from build123d import *

# Parameters (mm, degrees)
BOSS_EXTRU_2_DEPTH                 = 10
CONG_1_R                           = 0.45
R_P_TITION_CIRCULAIRE1_COUNT       = 8
R_P_TITION_CIRCULAIRE1_ANGLE       = 210
CONG_1_OF_R_P_TITION_CIRCULAIRE1_R = 0.45
ESQUISSE5_R                        = 7.125
BOSS_EXTRU_4_DEPTH                 = 10
ENL_V_MAT_EXTRU_3_DEPTH            = 11
ESQUISSE3_R                        = 1.6
ENL_V_MAT_EXTRU_4_DEPTH            = 11
ESQUISSE8_R                        = 1.6
ENL_V_MAT_EXTRU_5_DEPTH            = 11


with BuildPart() as part:
    # Esquisse1 → Boss.-Extru.2 (new body)
    with BuildSketch(Plane.XY):
        with BuildLine():
            Line((0, 0), (6.882221512, 1.844085696))
            ThreePointArc((6.882221512, 1.844085696), (6.988095123, 1.390018544), (7.064044637, 0.92999912))
            Line((7.064044637, 0.92999912), (8.384880781, 1.103890497))
            ThreePointArc((8.384880781, 1.103890497), (9.465680859, 1.068283463), (10.477518694, 0.686732857))
            ThreePointArc((10.477518694, 0.686732857), (10.5, 0), (10.477518694, -0.686732857))
            ThreePointArc((10.477518694, -0.686732857), (9.465680859, -1.068283463), (8.384880781, -1.103890497))
            Line((8.384880781, -1.103890497), (7.064044637, -0.92999912))
            ThreePointArc((7.064044637, -0.92999912), (6.988095123, -1.390018544), (6.882221512, -1.844085696))
            Line((6.882221512, -1.844085696), (0, 0))
        make_face()
    boss_extru_2 = extrude(amount=BOSS_EXTRU_2_DEPTH)

    # Congé1
    cong_1_edges = [part.edges().sort_by_distance(p)[0] for p in [
        (7.064044637, 0.92999912, 5),
        (7.064044637, -0.92999912, 5),
    ]]
    fillet(cong_1_edges, radius=CONG_1_R)

    # Répétition circulaire1: Boss.-Extru.2 ×8 about axis
    r_p_tition_circulaire1_axis = Axis((0, 0, 0), (0, 0, -1))
    for i in range(1, R_P_TITION_CIRCULAIRE1_COUNT):
        add(boss_extru_2.rotate(r_p_tition_circulaire1_axis, i * R_P_TITION_CIRCULAIRE1_ANGLE / (R_P_TITION_CIRCULAIRE1_COUNT - 1)))

    # Congé1 of Répétition circulaire1
    cong_1_of_r_p_tition_circulaire1_edges = [part.edges().sort_by_distance(p)[0] for p in [
        (6.582641669, -2.726619456, 5),
        (5.65264255, -4.337425182, 5),
        (4.337425182, -5.65264255, 5),
        (2.726619456, -6.582641669, 5),
        (0.92999912, -7.064044637, 5),
        (-0.92999912, -7.064044637, 5),
        (-2.726619456, -6.582641669, 5),
        (-4.337425182, -5.65264255, 5),
        (-5.65264255, -4.337425182, 5),
        (-6.582641669, -2.726619456, 5),
        (-7.064044637, -0.92999912, 5),
        (-7.064044637, 0.92999912, 5),
        (-6.582641669, 2.726619456, 5),
        (-5.65264255, 4.337425182, 5),
    ]]
    fillet(cong_1_of_r_p_tition_circulaire1_edges, radius=CONG_1_OF_R_P_TITION_CIRCULAIRE1_R)

    # Esquisse5 → Boss.-Extru.4 (add, through all)
    with BuildSketch(Plane.XY.offset(10)):
        Circle(ESQUISSE5_R)
    extrude(amount=-BOSS_EXTRU_4_DEPTH)

    # Esquisse7 → Enlèv. mat.-Extru.3 (cut, through all)
    with BuildSketch(Plane.XY.offset(10)):
        with BuildLine():
            Line((-3.608929902, 6.143390755), (6.197120353, 3.515867508))
            ThreePointArc((6.197120353, 3.515867508), (1.844085696, 6.882221512), (-3.608929902, 6.143390755))
        make_face()
    extrude(amount=-ENL_V_MAT_EXTRU_3_DEPTH, mode=Mode.SUBTRACT)

    # Esquisse3 → Enlèv. mat.-Extru.4 (cut, through all)
    with BuildSketch(Plane.XY.offset(10)):
        Circle(ESQUISSE3_R)
    extrude(amount=-ENL_V_MAT_EXTRU_4_DEPTH, mode=Mode.SUBTRACT)

    # Esquisse8 → Enlèv. mat.-Extru.5 (cut, through all)
    with BuildSketch(Plane.XY.offset(10)):
        with Locations((-4.330127019, 2.5)):
            Circle(ESQUISSE8_R)
        with Locations((4.330127019, -2.5)):
            Circle(ESQUISSE8_R)
    extrude(amount=-ENL_V_MAT_EXTRU_5_DEPTH, mode=Mode.SUBTRACT)


solid = part.part
Design review of the part built by this model. Coordinates are the model's own, in mm. A direction names the side the tool comes from. Give positions to 0.01 mm unless a question says otherwise; leave off trailing zeros. Loops run counter-clockwise (first coordinate to the right, second up) from the corner with the lowest first, then second, coordinate; pieces in that order, holes last. Notation, with made-up numbers: (-37, 50) -> (-31, 50) arc R19 ccw to (-31, 65) -> close; hole circle Ø6 at (-35.75, -7.5). An arc over 180 degrees is marked (long way). One line per question, with ' | ' between items. Start each with the question number.
(1) We need section D-D (z = 5). State how many separate pieces and enclosed holes the cut face has, and give its area (3 significant figures).
(2) We need section A-A (y = 0). State the section outline as (x, z) points, and give its area (3 significant figures).
(3) For faces 5 (the face through (5.653, -7.649, 4.93)), 6 (the face through (3.818, -8.743, 4.93)), 7 (the face through (9.481, -1.065, 4.93)), 8 (the face through (-5.663, -7.678, 4.93)), list the 3-axis set-ups (+Z, -Z, +X, -X, +Y, -Y) from which the entire face can be reached by the end or side of a thin tool; tool diameter is ignored.
(4) We need section B-B (x = -4). State the section outline as (y, z) points, and give its area (3 significant figures).
(5) Draft analysis for pull direction X (two halves, no side actions). For faces 1 (the face through (7.39, -3.06, 4.93)), 2 (the face through (-10.5, 0, 4.9)), 3 (the face through (-1, -2, 10)), 4 (the face through (-3.06, -7.39, 4.93)), state which applies: +X half, -X half, draft (parallel to the pull), parting line (faces both ways), or undercut.
(6) For line 1 (Y direction, x = -5, z = 3); line 2 (Y direction, x = -4.75, z = 6.5); line 3 (Y direction, x = 2.5, z = 5.75), list the stretches that pass through material, from the lowest coordinate up.
(7) We need section C-C (x = -7.25). State the section outline as (y, z) points, and give its area (3 significant figures).
(8) Insertion check: P1, Ø2.5, axis at x = 4.33, y = -2.5, coming from the -Z side; P2, Ø6, axis at y = -6, z = 8, coming from the -X side. Each pin has a flat end and moves straight along its axis. Give the tip position at first contact, or say it passes through.
The answers:
1) separate pieces: 1 | enclosed holes: 3 | area: 176 mm^2
2) outline: (-10.5, 0) -> (-1.6, 0) -> (-1.6, 10) -> (-10.5, 10) -> close; (1.6, 0) -> (10.5, 0) -> (10.5, 10) -> (1.6, 10) -> close | area: 178 mm^2
3) face 5: +Z, -Z, +X | face 6: +Z, -Z, -Y | face 7: +Z, -Z | face 8: +Z, -Z, -X
4) outline: (-8.93, 0) -> (0.93, 0) -> (0.93, 10) -> (-8.93, 10) -> close; (4.07, 0) -> (5.9, 0) -> (5.9, 10) -> (4.07, 10) -> close | area: 117 mm^2
5) face 1: +X half | face 2: -X half | face 3: draft | face 4: undercut
6) line 1: y = -9.23 to -6.52, -5.08 to 1.05, 3.95 to 5.08 | line 2: y = -9.36 to -6.19, -5.31 to 0.96, 4.04 to 5.31 | line 3: y = -6.71 to 4.51
7) outline: (-5.49, 0) -> (-3, 0) -> (-3, 10) -> (-5.49, 10) -> close; (-1.02, 0) -> (1.02, 0) -> (1.02, 10) -> (-1.02, 10) -> close; (3, 0) -> (5.49, 0) -> (5.49, 10) -> (3, 10) -> close | area: 70.1 mm^2
8) P1: passes through | P2: stops at x = -9.42
